Autodesk Inventor part; units mm, degrees
ref_plane "YZ Plane" through (0, 0, 0) normal (1, 0, 0) x (0, 1, 0)
ref_plane "XZ Plane" through (0, 0, 0) normal (0, 1, 0) x (-1, 0, 0)
ref_plane "XY Plane" through (0, 0, 0) normal (0, 0, 1) x (1, 0, 0)
sketch "Náčrt2" plane through (0, 0, 0) normal (0, 1, 0) x (-1, 0, 0)
  line L0 (11.5, 17.5) -> (-11.5, 17.5) construction
  line L1 (-17.5, 11.5) -> (-17.5, -11.5) construction
  line L2 (-11.5, -17.5) -> (11.5, -17.5) construction
  line L3 (17.5, -11.5) -> (17.5, 11.5) construction
  line L4 (42.5, 36) -> (42.5, -77.5) construction
  line L5 (9, -22.5) -> (-14, -22.5) construction
  line L6 (-20, -28.5) -> (-20, -51.5) construction
  line L7 (-14, -57.5) -> (9, -57.5) construction
  line L8 (15, -51.5) -> (15, -28.5) construction
  arc A0 (15, -28.5) -> (9, -22.5) centre (9, -28.5) ccw construction
  arc A1 (9, -57.5) -> (15, -51.5) centre (9, -51.5) ccw construction
  arc A2 (-20, -51.5) -> (-14, -57.5) centre (-14, -51.5) ccw construction
  arc A3 (-14, -22.5) -> (-20, -28.5) centre (-14, -28.5) ccw construction
  line L9 (-45.6938, -20) -> (9, -20) construction
  arc A4 (17.5, -28.5) -> (9, -20) centre (9, -28.5) ccw construction
  line L10 (17.5, -28.5) -> (17.5, -51.5) construction
  line L11 (17.5, -51.5) -> (15, -51.5) construction
  line L12 (-14, -22.5) -> (-45.6938, -22.5) construction
  line L13 (-45.6938, -22.5) -> (-45.6938, -20) construction
  arc A5 (17.5, 11.5) -> (11.5, 17.5) centre (11.5, 11.5) ccw construction
  arc A6 (11.5, -17.5) -> (17.5, -11.5) centre (11.5, -11.5) ccw construction
  arc A7 (-17.5, -11.5) -> (-11.5, -17.5) centre (-11.5, -11.5) ccw construction
  arc A8 (-11.5, 17.5) -> (-17.5, 11.5) centre (-11.5, 11.5) ccw construction
  line L14 (-11.5, -20) -> (11.5, -20) construction
  line L15 (-20, 73.4113) -> (-20, -11.5) construction
  arc A9 (-20, -11.5) -> (-11.5, -20) centre (-11.5, -11.5) ccw construction
  line L16 (-17.5, 11.5) -> (-17.5, 73.4113) construction
  line L17 (-17.5, 73.4113) -> (-20, 73.4113) construction
  line L18 (11.5, -20) -> (11.5, -17.5) construction
  line L19 (17.5, 17.5) -> (-17.5, 17.5) construction
  line L20 (-17.5, 17.5) -> (-17.5, 52.5) construction
  line L21 (-17.5, 52.5) -> (17.5, 52.5) construction
  line L22 (17.5, 52.5) -> (17.5, 17.5) construction
  circle A10 centre (0, 35) radius 6.5
  arc A11 (0, 51) -> (0, 19) centre (0, 35) ccw construction
  line L23 (0, 51) -> (27.5, 51) construction
  line L24 (0, 19) -> (11.5, 19) construction
  line L25 (27.5, 51) -> (42.5, 36) construction
  arc A12 (17.5, 13) -> (11.5, 19) centre (11.5, 13) ccw construction
  line L26 (17.5, 13) -> (17.5, -51.5) construction
  line L27 (-13.5, -57.5) -> (-13.5, -59.2574) construction
  line L28 (-12.6213, -61.3787) -> (14.1066, -88.1066) construction
  line L29 (24.7132, -92.5) -> (27.5, -92.5) construction
  arc A13 (27.5, -92.5) -> (42.5, -77.5) centre (27.5, -77.5) ccw construction
  arc A14 (14.1066, -88.1066) -> (24.7132, -92.5) centre (24.7132, -77.5) ccw construction
  arc A15 (-13.5, -59.2574) -> (-12.6213, -61.3787) centre (-10.5, -59.2574) ccw construction
  line L30 (17.5, -51.5) -> (17.5, -51.5) construction
  line L31 (6.4677, -58.2408) -> (-10.5, -57.5) construction
  line L32 (-13.5, -57.5) -> (-10.5, -57.5) construction
  line L33 (6.4677, -58.2408) -> (6.5, -57.5) construction
  line L34 (6.5, -57.5) -> (11.5, -57.5) construction
  arc A16 (11.5, -57.5) -> (17.5, -51.5) centre (11.5, -51.5) ccw construction
  arc A17 (-16, 35) -> (16, 35) centre (0, 35) ccw
  line L35 (16, 35) -> (16, 87)
  line L36 (-16, 35) -> (-16, 99)
  line L37 (24, 139) -> (94, 139)
  line L38 (104, 129) -> (104, 117)
  line L39 (94, 107) -> (36, 107)
  arc A18 (36, 107) -> (16, 87) centre (36, 87) ccw
  arc A19 (24, 139) -> (-16, 99) centre (24, 99) ccw
  arc A20 (104, 129) -> (94, 139) centre (94, 129) ccw
  arc A21 (94, 107) -> (104, 117) centre (94, 117) ccw
  point P0 (0, 0)
  point P1 (17.5, 0)
  point P2 (0, 17.5)
  point P3 (42.5, 51)
  point P4 (17.5, 35)
  point P5 (0, 52.5)
  point P6 (-13.5, -60.5)
  point P7 (16, 107)
  point P8 (-16, 139)
  point P9 (104, 139)
  point P10 (104, 107)
  dimension "d34" = 35
  dimension "d35" = 6
  dimension "d36" = 5
  dimension "d37" = 2.5
  dimension "d38" = 2.5
  dimension "d39" = 6
  dimension "d40" = 2.5
  dimension "d43" = 25
  dimension "d46" = 13
  dimension "d47" = 32
  dimension "d48" = 15
  dimension "d49" = 15
  dimension "d50" = 6
  dimension "d51" = 35
  dimension "d55" = 3
  dimension "d56" = 15
  dimension "d57" = 15
  dimension "d58" = 3
  dimension "d60" = 35
  dimension "d61" = 3
  dimension "d62" = 2.5
  dimension "d63" = 35
  dimension "d64" = 45
  dimension "d66" = 31
  dimension "d69" = 6
  dimension "d72" = 2.5
  dimension "d79" = 32
  dimension "d80" = 120
  dimension "d81" = 120
  dimension "d82" = 20
  dimension "d83" = 40
  dimension "d85" = 10
extrude "Vysunutí1" add sketch "Náčrt2" along normal blind 6
sketch "Náčrt5" plane through (0, 0, 0) normal (0, -1, 0) x (1, 0, 0)
  circle A0 centre (0, 35) radius 6.5
  arc A1 (-16, 35) -> (16, 35) centre (0, 35) ccw
  line L0 (16, 99) -> (16, 35)
  line L1 (-16, 35) -> (-16, 87)
  circle A2 centre (-88, 123) radius 5
  arc A3 (16, 99) -> (-24, 139) centre (-24, 99) ccw
  line L2 (-94, 139) -> (-24, 139)
  line L3 (-104, 117) -> (-104, 129)
  line L4 (-36, 107) -> (-94, 107)
  arc A4 (-16, 87) -> (-36, 107) centre (-36, 87) ccw
  arc A5 (-94, 139) -> (-104, 129) centre (-94, 129) ccw
  arc A6 (-104, 117) -> (-94, 107) centre (-94, 117) ccw
  point P0 (0, 0)
  point P1 (-104, 123)
  dimension "d75" = 10
  dimension "d84" = 16
extrude "Vysunutí3" cut sketch "Náčrt5" against normal blind 10 contours A2
fillet "Zaoblení6" radius 3 2 edges at (-93, 0, 123) (-93, 6, 123)
equation "\"d79\" = d47"
equation "\"d81\" = d80"
equation "\"PoloměrOhybu\" = Tloušťka"
equation "\"ŠířkaVýštipu\" = Tloušťka"
equation "\"HloubkaVýštipu\" = 0.5 * Tloušťka"
equation "\"VelikostRohovéhoVýštipu\" = 4 * Tloušťka"
equation "\"MinimálníZbytek\" = 2 * Tloušťka"
equation "\"PřechodovýPoloměr\" = PoloměrOhybu"
equation "\"VelikostJacobihoPoloměru\" = PoloměrOhybu"
equation "\"VelikostMezery\" = Tloušťka"
properties part number "DD_KVD_002_10" material "Nerezová ocel"
Part model, mm, in its own coordinate system. A direction names the side the tool comes from. Coordinates: 2 decimals unless noted, no trailing zeros. Write each loop counter-clockwise with the first axis right and the second up, starting at its lowest first coordinate (ties: lowest second). Pieces come first, ordered by that corner, then holes. Notation, with made-up numbers: (-2.75, 11) - (11.25, 11) arc R18 cw to (11.25, 30) - close; hole circle Ø5 at (21.5, 64.5). An arc over 180 degrees is marked (long way). Put each result on its own line as item: value.
1. 3-axis set-ups, long thin cutter, end or side, ignore diameter. For faces 1 (the flat face through (-16, 3, 61)), 2 (the flat face through (16, 3, 67)): which of +Z, -Z, +X, -X, +Y, -Y reach the whole face in a straight line?
Final values:
face 1: -Z, -X, +Y, -Y
face 2: +Z, -Z, +X, +Y, -Y
2. Probe line 1 along Z through (x, y) = (0, 3.6); line 2 along Z through (x, y) = (-88, 3.05); line 3 along X through (y, z) = (3.05, 123). List the from-to ranges inside material, lowest first. Write a range as [from, to].
Final values:
line 1: z = [19, 28.5], [41.5, 131]
line 2: z = [107, 118], [128, 139]
line 3: x = [-104, -93], [-83, 8]
3. Flat gauge pins, fed straight in: pin 1 Ø13 at (x, z) = (-88, 123) entering from +Y; pin 2 Ø11.5 at (x, z) = (0, 35) entering from -Y; pin 3 Ø3 at (x, y) = (-53, 2.5) entering from -Z; pin 4 Ø1 at (y, z) = (4.5, 97.5) entering from -X. Where does each tip first touch, or does it go through?
Final values:
pin 1: stops at y = 5.6
pin 2: passes through
pin 3: stops at z = 107
pin 4: stops at x = -19.3
4. Two-plate mould, pull along Z, no slides. Class faces 3 (the flat face through (-16, 0, 93)), 4 (the cylindrical face through (0, 3, 19)), 5 (the cylindrical face through (0.846, 2.958, 28.555)), 6 (the cylindrical face through (4.594, 2.958, 126.972)): +Z half, -Z half, draft (parallel to the pull), parting line (faces both ways), or undercut.
Final values:
face 3: draft
face 4: -Z half
face 5: undercut
face 6: +Z half
5. Band-saw the part on D-D (x = 0). Write the cut outline in (y, z), then the cut area to 3 significant figures.
Final values:
outline: (0, 19) - (6, 19) - (6, 28.5) - (0, 28.5) - close; (0, 41.5) - (6, 41.5) - (6, 131) - (0, 131) - close
area: 594 mm²
6. Band-saw the part on C-C (y = 4.65). Write the cut outline in (x, z).
Final values:
outline: (-104, 117) arc R10 ccw to (-94, 107) - (-36, 107) arc R20 cw to (-16, 87) - (-16, 35) arc R16 ccw to (16, 35) - (16, 99) arc R40 ccw to (-24, 139) - (-94, 139) arc R10 ccw to (-104, 129) - close; hole circle Ø10.99 at (-88, 123); hole circle Ø13 at (0, 35)
